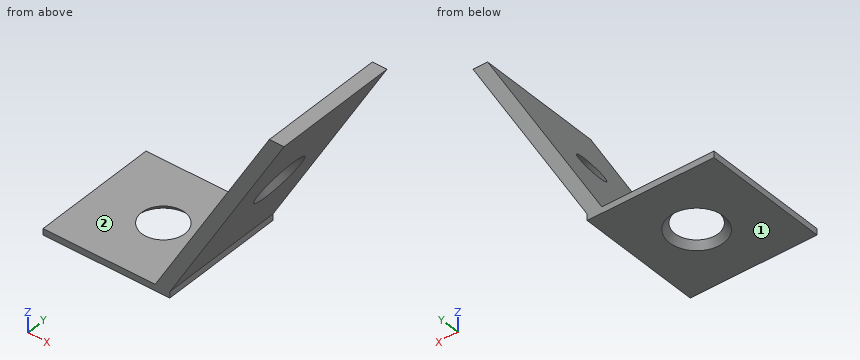
```python
from build123d import *

# Parameters (mm, degrees)
SKETCH2_W                                         = 10
SKETCH2_H                                         = 10
BOSS_EXTRUDE1_DEPTH                               = 0.5
BOSS_EXTRUDE2_DEPTH                               = 10
CSK_FOR_1_FLAT_HEAD_SOCKET_CAP_SCREW1_D           = 2.0574
CSK_FOR_1_FLAT_HEAD_SOCKET_CAP_SCREW1_CSINK_D     = 4.2672
CSK_FOR_1_FLAT_HEAD_SOCKET_CAP_SCREW1_CSINK_ANGLE = 82
CSK_FOR_1_FLAT_HEAD_SOCKET_CAP_SCREW2_D           = 2.0574
CSK_FOR_1_FLAT_HEAD_SOCKET_CAP_SCREW2_CSINK_D     = 4.2672
CSK_FOR_1_FLAT_HEAD_SOCKET_CAP_SCREW2_CSINK_ANGLE = 82


with BuildPart() as part:
    # Sketch2 → Boss-Extrude1 (new body)
    with BuildSketch(Plane.XY):
        with Locations((5, -5)):
            Rectangle(SKETCH2_W, SKETCH2_H)
    extrude(amount=BOSS_EXTRUDE1_DEPTH)

    # Sketch3 → Boss-Extrude2 (add)
    with BuildSketch(Plane.XZ.offset(10)):
        Polygon((8.845299462, 0.5), (17.845299462, 16.088457268), (19, 16.088457268), (10, 0.5), align=None)
    extrude(amount=-BOSS_EXTRUDE2_DEPTH)

    # CSK for #1 Flat Head Socket Cap Screw1 (through all)
    with Locations(Plane(origin=(0, 0, 0), x_dir=(-1, 0, 0), z_dir=(0, 0, -1))):
        with Locations((-5.362516401, -4.921292394)):
            CounterSinkHole(CSK_FOR_1_FLAT_HEAD_SOCKET_CAP_SCREW1_D / 2, CSK_FOR_1_FLAT_HEAD_SOCKET_CAP_SCREW1_CSINK_D / 2, counter_sink_angle=CSK_FOR_1_FLAT_HEAD_SOCKET_CAP_SCREW1_CSINK_ANGLE)

    # CSK for #1 Flat Head Socket Cap Screw2 (through all)
    with Locations(Plane(origin=(7.283493649, 0, -4.205127019), x_dir=(-0.5, 0, -0.866025404), z_dir=(0.866025404, 0, -0.5))):
        with Locations((-14.39146791, -4.879407471)):
            CounterSinkHole(CSK_FOR_1_FLAT_HEAD_SOCKET_CAP_SCREW2_D / 2, CSK_FOR_1_FLAT_HEAD_SOCKET_CAP_SCREW2_CSINK_D / 2, counter_sink_angle=CSK_FOR_1_FLAT_HEAD_SOCKET_CAP_SCREW2_CSINK_ANGLE)


solid = part.part
```
Could you check a few things on this model? Use its own coordinates, in mm. Face numbers are marked on the shaded views. A direction names the side the tool comes from. Round coordinates to 2 decimals unless told otherwise and drop trailing zeros. Loops run counter-clockwise (first coordinate to the right, second up) from the corner with the lowest first, then second, coordinate; pieces in that order, holes last. Notation, with made-up numbers: (67, -2) - (120, -2) arc R14 ccw to (120, 23) - close; hole circle Ø2 at (56.25, -39.5). An arc over 180 degrees is marked (long way). Answer in a Markdown table with one row per item. Add a question column.
(1) I need wall thicknesses on line 1 along Z through (x, y) = (4.25, -0.5); line 2 along X through (y, z) = (-3, 9.25); line 3 along X through (y, z) = (-8.5, 4.5). Which ranges of each line are inside material? Lowest first, please.
(2) If we section it at D-D (z = 5.5): Please give me the cut outline in (x, y).
(3) If we section it at B-B (x = 1.75): Please give me the cut outline in (y, z), plus the area to 3 significant figures.
(4) I'm going to push flat-ended pins straight in: pin 1 (6 mm diameter, centred on x = 3.5, y = -6, fed in from +Z); pin 2 (1 mm diameter, centred on y = -7.5, z = 7, fed in from -X); pin 3 (5 mm diameter, centred on y = -2.5, z = 10.5, fed in from +X). Where does each tip first touch, or does it pass through?
(5) If we section it at A-A (y = -2.25): Please give me the cut outline in (x, z).
(6) If we section it at C-C (y = -4.5): State how many separate pieces and enclosed holes the cut face has, plus the area to 3 significant figures.
(7) For the marked faces 1 and 2, which set-ups out of +Z, -Z, +X, -X, +Y, -Y let a thin tool reach every point of the face, with its end or its side?
Model answer:
| question | item | result |
|---|---|---|
| 1 | line 1 | z = 0 to 0.5 |
| 1 | line 2 | x = 13.9 to 15.05 |
| 1 | line 3 | x = 11.15 to 12.31 |
| 2 | outline | (11.73, -10) - (12.89, -10) - (12.89, 0) - (11.73, 0) - close |
| 3 | outline | (-10, 0) - (0, 0) - (0, 0.5) - (-10, 0.5) - close |
| 3 | area | 5.00 mm² |
| 4 | pin 1 | stops at z = 0.5 |
| 4 | pin 2 | stops at x = 12.31 |
| 4 | pin 3 | stops at x = 17.22 |
| 5 | outline | (0, 0) - (10, 0) - (10, 0.5) - (19, 16.09) - (17.85, 16.09) - (8.85, 0.5) - (0, 0.5) - close |
| 6 | separate pieces | 3 |
| 6 | enclosed holes | 0 |
| 6 | area | 17.8 mm² |
| 7 | face 1 | -Z, +X, -X, +Y, -Y |
| 7 | face 2 | +Z, -X, +Y, -Y |
